Source: CAD feature listing. Evaluate the final solid. Frame: model axes, mm. Give positions to 0.01 mm unless a question says otherwise; leave off trailing zeros. Loops run counter-clockwise (first coordinate to the right, second up) from the corner with the lowest first, then second, coordinate; pieces in that order, holes last. Notation, with made-up numbers: M 22.25,-35.75 L 52.25,-35.75 A31 cw 52.25,-2.75 Z; hole C 44,-40 d11. An arc over 180 degrees is marked long. Answer in a Markdown table with one row per item.
```python
from build123d import *

# Parameters (mm, degrees)
SKETCH4_W                    = 140
SKETCH4_H                    = 30
BOSS_EXTRUDE2_DEPTH          = 5
SKETCH5_R                    = 5.5
CUT_EXTRUDE1_DEPTH           = 63
M16_TAPPED_HOLE1_D           = 14
M16_TAPPED_HOLE1_DEPTH       = 38
M16_TAPPED_HOLE1_CSINK_D     = 16.05
M16_TAPPED_HOLE1_CSINK_ANGLE = 90
M16_TAPPED_HOLE1_TIP         = 4.206024333


with BuildPart() as part:
    # Sketch4 → Boss-Extrude2 (new, symmetric)
    with BuildSketch(Plane(origin=(0, 0, 0), x_dir=(1, 0, 0), z_dir=(0, 1, 0))):
        Rectangle(SKETCH4_W, SKETCH4_H)
    extrude(amount=BOSS_EXTRUDE2_DEPTH, both=True)

    # Sketch5 → Cut-Extrude1 (cut)
    with BuildSketch(Plane(origin=(0, 5, 0), x_dir=(1, 0, 0), z_dir=(0, 1, 0))):
        with Locations(Location((-60, 0, 0), (0, 0, 270))):
            Circle(SKETCH5_R)
        with Locations(Location((60, 0, 0), (0, 0, 270))):
            Circle(SKETCH5_R)
    extrude(amount=-CUT_EXTRUDE1_DEPTH, mode=Mode.SUBTRACT)

    # M16 Tapped Hole1
    with Locations(Plane.ZX.offset(5)):
        with Locations((0, 0)):
            CounterSinkHole(M16_TAPPED_HOLE1_D / 2, M16_TAPPED_HOLE1_CSINK_D / 2, depth=M16_TAPPED_HOLE1_DEPTH, counter_sink_angle=M16_TAPPED_HOLE1_CSINK_ANGLE)
            with Locations((0, 0, -(M16_TAPPED_HOLE1_DEPTH + M16_TAPPED_HOLE1_TIP / 2))):  # 118° drill point
                Cone(0, M16_TAPPED_HOLE1_D / 2, M16_TAPPED_HOLE1_TIP, mode=Mode.SUBTRACT)


solid = part.part
```
1) Pull-direction query (Z, two-part tool) for faces 1 (the flat face through (70, 0, 0)), 2 (the cylindrical face through (65.453, 0.07, -0.716)), 3 (the flat face through (-1, 0, 15)), 4 (the cylindrical face through (-54.547, 0.07, -0.716)); classes: released by +Z, released by -Z, zero draft, split by the parting line, or undercut.
Reply:
| item | result |
|---|---|
| face 1 | zero draft |
| face 2 | undercut |
| face 3 | released by +Z |
| face 4 | undercut |
2) Section B-B, the plane z = 0. Return loops of the section in (x, y) (3 decimals), then the cut area to 3 significant figures.
Reply:
| item | result |
|---|---|
| outline | M -70,-5 L -65.5,-5 L -65.5,5 L -70,5 Z; M -54.5,-5 L -7,-5 L -7,3.975 L -8.025,5 L -54.5,5 Z; M 7,-5 L 54.5,-5 L 54.5,5 L 8.025,5 L 7,3.975 Z; M 65.5,-5 L 70,-5 L 70,5 L 65.5,5 Z |
| area | 1,040 mm² |
3) Section C-C, the plane y = 2. Return loops of the section in (x, z).
Reply:
| item | result |
|---|---|
| outline | M -70,-15 L 70,-15 L 70,15 L -70,15 Z; hole C -60,0 d11; hole C 0,0 d14; hole C 60,0 d11 |
4) Material intervals for L1, parallel to X at y = 1.5, z = 0; L2, parallel to X at y = -2.5, z = -2.75; L3, parallel to Z at x = 0, y = -0.5, sorted ascending.
Reply:
| item | result |
|---|---|
| L1 | x = -70 to -65.5, -54.5 to -7, 7 to 54.5, 65.5 to 70 |
| L2 | x = -70 to -64.76, -55.24 to -6.44, 6.44 to 55.24, 64.76 to 70 |
| L3 | z = -15 to -7, 7 to 15 |
5) Section A-A, the plane x = -60. Return loops of the section in (y, z).
Reply:
| item | result |
|---|---|
| outline | M -5,-15 L 5,-15 L 5,-5.5 L -5,-5.5 Z; M -5,5.5 L 5,5.5 L 5,15 L -5,15 Z |
